```python
from build123d import *

# Parameters (mm, degrees)
BOSS_EXTRUDE2_DEPTH = 40
SKETCH2_W           = 40
SKETCH2_H           = 30
CUT_EXTRUDE1_DEPTH  = 30
SKETCH3_R           = 5
BOSS_EXTRUDE3_DEPTH = 30
SKETCH4_W           = 80
SKETCH4_H           = 30
CUT_EXTRUDE2_DEPTH  = 30
SKETCH5_R           = 5
BOSS_EXTRUDE4_DEPTH = 30


with BuildPart() as part:
    # Sketch1 → Boss-Extrude2 (new body)
    with BuildSketch(Plane.XY):
        Polygon((106.666666667, 22.215384615), (106.666666667, 62.215384615), (-53.333333333, 62.215384615), (-53.333333333, -107.008547009), (15.753846154, -211.2), (90.584615385, -237.784615385), (6.666666667, -107.008547009), (6.666666667, 22.215384615), align=None)
    extrude(amount=BOSS_EXTRUDE2_DEPTH)

    # Sketch2 → Cut-Extrude1 (cut)
    with BuildSketch(Plane(origin=(0, 62.215384615, 0), x_dir=(1, 0, 0), z_dir=(0, 1, 0))):
        with Locations((-33.333333333, -20)):
            Rectangle(SKETCH2_W, SKETCH2_H)
    extrude(amount=-CUT_EXTRUDE1_DEPTH, mode=Mode.SUBTRACT)

    # Sketch3 → Boss-Extrude3 (add)
    with BuildSketch(Plane.XY.offset(5)):
        with Locations(Location((-38.333333333, 47.215384615, 0), (0, 0, 180))):
            Circle(SKETCH3_R)
    extrude(amount=BOSS_EXTRUDE3_DEPTH)

    # Sketch4 → Cut-Extrude2 (cut)
    with BuildSketch(Plane(origin=(0, 62.215384615, 0), x_dir=(1, 0, 0), z_dir=(0, 1, 0))):
        with Locations((66.666666667, -20)):
            Rectangle(SKETCH4_W, SKETCH4_H)
    extrude(amount=-CUT_EXTRUDE2_DEPTH, mode=Mode.SUBTRACT)

    # Sketch5 → Boss-Extrude4 (add)
    with BuildSketch(Plane.XY.offset(5)):
        with Locations(Location((91.666666667, 47.215384615, 0), (0, 0, 180))):
            Circle(SKETCH5_R)
    extrude(amount=BOSS_EXTRUDE4_DEPTH)


solid = part.part
```
Check sheet for the modelled part. Datum: model origin and axes. Units: mm. A direction names the side the tool comes from. Round coordinates to 2 decimals unless told otherwise and drop trailing zeros. Write each loop counter-clockwise with the first axis right and the second up, starting at its lowest first coordinate (ties: lowest second). Pieces come first, ordered by that corner, then holes. Notation, with made-up numbers: (-23.75, 72.25) -> (35.25, 72.25) arc R18 cw to (35.25, 104.25) -> close; hole circle Ø4 at (-19, 9). An arc over 180 degrees is marked (long way). One line per question, with ' | ' between items. Start each with the question number.
1. Release check for a two-part mould opening along Z. For faces 1 (the face through (66, 32.215, 20)), 2 (the face through (-34, 44, 35)), 3 (the face through (6.667, -43, 20)), 4 (the face through (-10, -52, 0)) record: +Z half, -Z half, draft (parallel to the pull), parting line (faces both ways), or undercut.
2. Depth check by flat-ended pin: pin 1 (20 mm diameter, centred on y = -34, z = 23.5, fed in from +X); pin 2 (9 mm diameter, centred on x = -25, z = 18, fed in from +Y); pin 3 (24 mm diameter, centred on y = 45, z = 13, fed in from -X); pin 4 (12 mm diameter, centred on x = 82.5, z = 20, fed in from -Y). Enter the tip coordinate at first touch or a pass-through.
3. Sectioned sample at B-B, the plane z = 9. Record the cut outline in (x, y).
4. Set-up check for faces 5 (the face through (49.21, -173.31, 19.72)), 6 (the face through (-42.952, 49.13, 19.79)), 7 (the face through (-13.333, 47, 20)): record each of +Z, -Z, +X, -X, +Y, -Y from which the full face is reachable in a straight line by a thin tool's end or side.
5. Sectioned sample at A-A, the plane x = 72. Record the cut outline in (y, z).
6. Scan lines: line 1 along Z through (x, y) = (60, 33); line 2 along X through (y, z) = (49, 21.5); line 3 along X through (y, z) = (-67.5, 26.5). Record each from-to range of solid material in increasing order. Write a range as from..to.
7. Sectioned sample at C-C, the plane x = -39. Record the cut outline in (y, z), then the cut area to 3 significant figures.
8. Sectioned sample at D-D, the plane y = -59.5. Record the cut outline in (x, z).
Taken from the geometry:
1) face 1: undercut | face 2: undercut | face 3: draft | face 4: -Z half
2) pin 1: stops at x = 6.67 | pin 2: stops at y = 32.22 | pin 3: stops at x = -53.33 | pin 4: stops at y = -237.04
3) outline: (-53.33, -107.01) -> (15.75, -211.2) -> (90.58, -237.78) -> (6.67, -107.01) -> (6.67, 22.22) -> (106.67, 22.22) -> (106.67, 32.22) -> (26.67, 32.22) -> (26.67, 62.22) -> (-13.33, 62.22) -> (-13.33, 32.22) -> (-53.33, 32.22) -> close; circle Ø10 at (-38.33, 47.22); circle Ø10 at (91.67, 47.22)
4) face 5: +Z, -Z, +X | face 6: none | face 7: +Y
5) outline: (-231.18, 0) -> (-208.82, 0) -> (-208.82, 40) -> (-231.18, 40) -> close; (22.22, 0) -> (62.22, 0) -> (62.22, 5) -> (32.22, 5) -> (32.22, 35) -> (62.22, 35) -> (62.22, 40) -> (22.22, 40) -> close
6) line 1: z = 0..5, 35..40 | line 2: x = -43..-33.66, -13.33..26.67, 87..96.34 | line 3: x = -53.33..6.67
7) outline: (-128.62, 0) -> (62.22, 0) -> (62.22, 5) -> (52.17, 5) -> (52.17, 35) -> (62.22, 35) -> (62.22, 40) -> (-128.62, 40) -> close; hole (32.22, 5) -> (42.26, 5) -> (42.26, 35) -> (32.22, 35) -> close | area: 7,030 mm^2
8) outline: (-53.33, 0) -> (6.67, 0) -> (6.67, 40) -> (-53.33, 40) -> close
